Input: part model. Units: mm. Frame: model coordinates. A direction names the side the tool comes from. Coordinates: 2 decimals unless noted, no trailing zeros. Order: outer loops, then holes, each group sorted by start corner. A loop starts at its lowest first (then second) coordinate and runs counter-clockwise, first axis right, second up. Notation, with made-up numbers: (66, 57) - (125, 57) arc R12 ccw to (125, 70) - close; hole circle Ø9 at (40, -11). An arc over 180 degrees is marked (long way). Use a Markdown table: item, result. Add a question column.
from build123d import *

# Parameters (mm, degrees)
SKETCH1_R               = 27.94
BOSS_EXTRUDE1_DEPTH     = 3.175
SKETCH2_R               = 14.2875
BOSS_EXTRUDE2_DEPTH     = 9.525
CHAMFER1_SIZE           = 0.635
CUT_EXTRUDE2_DEPTH      = 1
CUT_EXTRUDE2_DEPTH_BACK = 13.7
SKETCH4_R               = 2.54
CUT_EXTRUDE3_DEPTH      = 13.7


with BuildPart() as part:
    # Sketch1 → Boss-Extrude1 (new body)
    with BuildSketch(Plane(origin=(0, 0, 0), x_dir=(1, 0, 0), z_dir=(0, 1, 0))):
        Circle(SKETCH1_R)
    extrude(amount=BOSS_EXTRUDE1_DEPTH)

    # Sketch2 → Boss-Extrude2 (add)
    with BuildSketch(Plane(origin=(0, 3.175, 0), x_dir=(1, 0, 0), z_dir=(0, 1, 0))):
        Circle(SKETCH2_R)
    extrude(amount=BOSS_EXTRUDE2_DEPTH)

    # Chamfer1
    chamfer1_edges = [part.edges().sort_by_distance(p)[0] for p in [
        (-14.2875, 12.7, 0),
    ]]
    chamfer(chamfer1_edges, length=CHAMFER1_SIZE)

    # Sketch3 → Cut-Extrude2 (cut, two sides)
    with BuildSketch(Plane(origin=(0, 12.7, 0), x_dir=(1, 0, 0), z_dir=(0, 1, 0))) as cut_extrude2_sk:
        Polygon((6.35, 3.666174209), (0, 7.332348419), (-6.35, 3.666174209), (-6.35, -3.666174209), (0, -7.332348419), (6.35, -3.666174209), align=None)
    extrude(amount=CUT_EXTRUDE2_DEPTH, mode=Mode.SUBTRACT)
    extrude(cut_extrude2_sk.sketch, amount=-CUT_EXTRUDE2_DEPTH_BACK, mode=Mode.SUBTRACT)

    # Sketch4 → Cut-Extrude3 (cut, through all)
    with BuildSketch(Plane.XZ):
        with Locations((0, 23.8125)):
            Circle(SKETCH4_R)
        with Locations((20.622229928, 11.90625)):
            Circle(SKETCH4_R)
        with Locations((20.622229928, -11.90625)):
            Circle(SKETCH4_R)
        with Locations((0, -23.8125)):
            Circle(SKETCH4_R)
        with Locations((-20.622229928, -11.90625)):
            Circle(SKETCH4_R)
        with Locations((-20.622229928, 11.90625)):
            Circle(SKETCH4_R)
    extrude(amount=-CUT_EXTRUDE3_DEPTH, mode=Mode.SUBTRACT)


solid = part.part
1) Contact query for flat-ended pins moving along their axis: P1, Ø6, axis at y = 2, z = -8.5, coming from the -X side; P2, Ø5, axis at x = 7, z = -18.5, coming from the +Y side (3 decimals); P3, Ø5, axis at y = 2.5, z = -19.5, coming from the -X side. Output: stop coordinate, or through.
2) Pull-direction query (X, two-part tool) for faces 4 (the flat face through (-3.219, 6.439, 5.474)), 5 (the cylindrical face through (-14.274, 7.558, -0.628)), 6 (the cylindrical face through (1.172, 1.565, -26.066)), 7 (the flat face through (3, 12.7, 6)); classes: pulls with the +X half, pulls with the -X half, needs draft (parallel to the pull), parting line crosses it, or undercut.
3) Reachability of faces 1 (the flat face through (-7, 0, 0)), 2 (the flat face through (3.131, 6.439, 5.525)), 3 (the flat face through (-7, 3.175, -13)) from +Z, -Z, +X, -X, +Y, -Y: full face, straight path, thin tool, end or side. Return the list, or none.
4) Cut plane C-C (x = -22.5). Return the cut outline in (y, z) (3 decimals), and give its area (3 significant figures).
5) Material intervals for L1, parallel to Z at x = 0, y = 2.55; L2, parallel to Y at x = 7.5, z = -23 (3 decimals); L3, parallel to X at y = 11, z = 3.5, sorted ascending.
6) Cut plane D-D (z = 11). State how many separate pieces and enclosed holes the cut face has, and give its area (3 significant figures).
Computed:
| question | item | result |
|---|---|---|
| 1 | P1 | stops at x = -27.39 |
| 1 | P2 | stops at y = 3.175 |
| 1 | P3 | stops at x = -22.17 |
| 2 | face 4 | undercut |
| 2 | face 5 | parting line crosses it |
| 2 | face 6 | undercut |
| 2 | face 7 | needs draft |
| 3 | face 1 | +Z, -Z, +X, -X, -Y |
| 3 | face 2 | +Y, -Y |
| 3 | face 3 | +Y |
| 4 | outline | (0, -16.565) - (3.175, -16.565) - (3.175, -13.617) - (0, -13.617) - close; (0, -10.196) - (3.175, -10.196) - (3.175, 10.196) - (0, 10.196) - close; (0, 13.617) - (3.175, 13.617) - (3.175, 16.565) - (0, 16.565) - close |
| 4 | area | 83.5 mm2 |
| 5 | L1 | z = -27.94 to -26.35, -21.27 to -7.33, 7.33 to 21.27, 26.35 to 27.94 |
| 5 | L2 | y = 0 to 3.175 |
| 5 | L3 | x = -13.85 to -6.35, 6.35 to 13.85 |
| 6 | separate pieces | 3 |
| 6 | enclosed holes | 0 |
| 6 | area | 306 mm2 |
